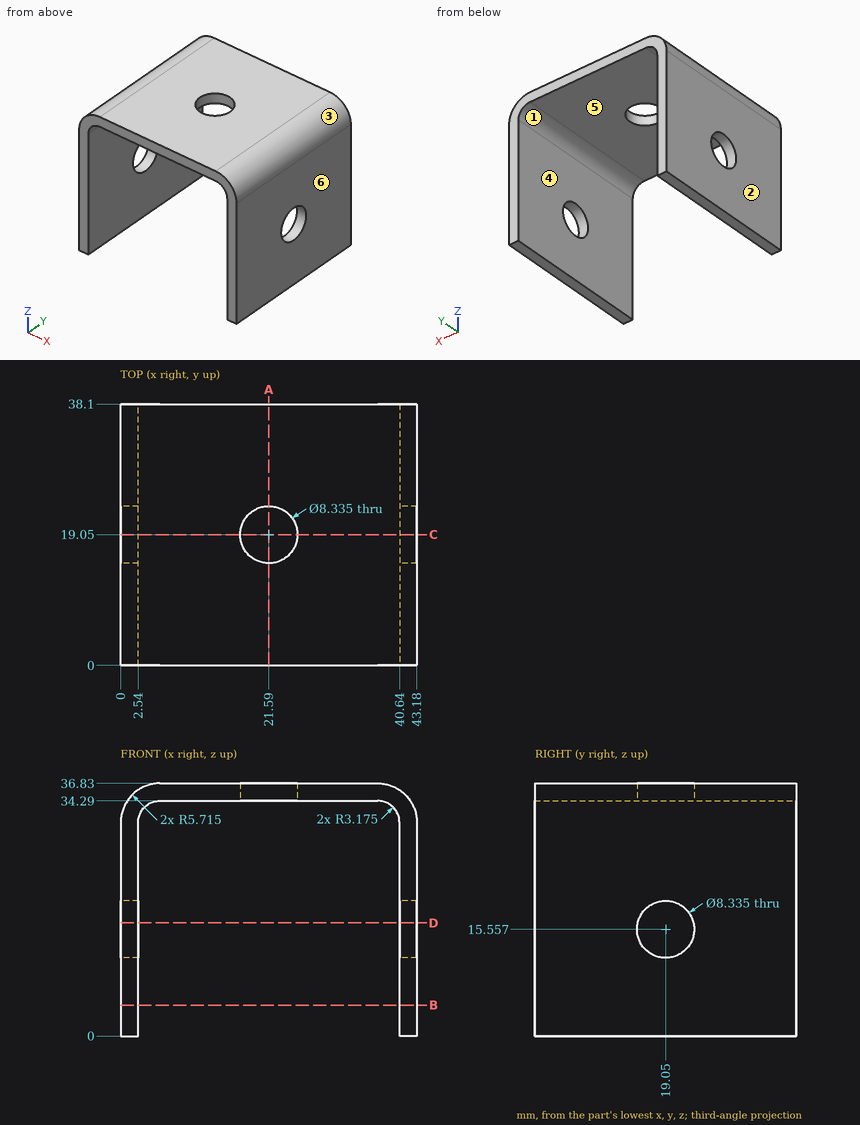
Check sheet for the drawn part. Datum: minimum x, y, z corner. Units: mm. A direction names the side the tool comes from. Round coordinates to 2 decimals unless told otherwise and drop trailing zeros. Loops run counter-clockwise (first coordinate to the right, second up) from the corner with the lowest first, then second, coordinate; pieces in that order, holes last. Notation, with made-up numbers: M 26.5,62.25 L 68.5,62.25 A20 ccw 68.5,91.25 Z; hole C 71.25,38 d6. An arc over 180 degrees is marked long. One line per question, with ' | ' between items. Start each with the question number.
Item 1: Section check C-C (y = 19.05). State how many separate pieces and enclosed holes the cut face has.
Item 2: Release check for a two-part mould opening along X. For the marked faces 1, 2, 3 and 4 record: released by +X, released by -X, zero draft, split by the parting line, or undercut.
Item 3: Scan lines: probe 1 along X at (y, z) = (5, 10.5); probe 2 along Z at (x, y) = (37.5, 23); probe 3 along Z at (x, y) = (1, 19) (1 decimal). Record each from-to range of solid material in increasing order.
Item 4: Set-up check for the marked faces 5 and 6: record each of +Z, -Z, +X, -X, +Y, -Y from which the full face is reachable in a straight line by a thin tool's end or side.
Item 5: Section check B-B (z = 4.5). Record the boundary of the cut face in (x, y).
Item 6: Section check A-A (x = 21.59). Record the boundary of the cut face in (y, z).
Item 7: Section check D-D (z = 16.5). Record the boundary of the cut face in (x, y), and give its area (3 significant figures).
Item 8: Gauge pin test, flat end, axial feed: pin 1 Ø3 at (x, y) = (21.5, 8.5) entering from -Z. Record the tip position at first contact, or that the pin passes through.
Worked out:
1) separate pieces: 4 | enclosed holes: 0
2) face 1: undercut | face 2: released by -X | face 3: released by +X | face 4: undercut
3) probe 1: 0 to 2.54, 40.64 to 43.18 | probe 2: 34.29 to 36.83 | probe 3: 0 to 11.4, 19.7 to 34.3
4) face 5: -Z, +Y, -Y | face 6: +Z, -Z, +X, +Y, -Y
5) outline: M 0,0 L 2.54,0 L 2.54,38.1 L 0,38.1 Z; M 40.64,0 L 43.18,0 L 43.18,38.1 L 40.64,38.1 Z
6) outline: M 0,34.29 L 14.88,34.29 L 14.88,36.83 L 0,36.83 Z; M 23.22,34.29 L 38.1,34.29 L 38.1,36.83 L 23.22,36.83 Z
7) outline: M 0,0 L 2.54,0 L 2.54,14.99 L 0,14.99 Z; M 0,23.11 L 2.54,23.11 L 2.54,38.1 L 0,38.1 Z; M 40.64,0 L 43.18,0 L 43.18,14.99 L 40.64,14.99 Z; M 40.64,23.11 L 43.18,23.11 L 43.18,38.1 L 40.64,38.1 Z | area: 152 mm^2
8) pin 1: z = 34.29
